The listing builds one solid part. Answer for the finished solid, in the listing's coordinates (mm). Give positions to 0.01 mm unless a question says otherwise; leave off trailing zeros. Order: outer loops, then holes, each group sorted by start corner. A loop starts at its lowest first (then second) coordinate and runs counter-clockwise, first axis right, second up. Notation, with made-up numbers: (6.5, 2) - (35.5, 2) arc R21 ccw to (35.5, 36) - close; hole circle Ø8 at (-25.5, 53.5). An arc over 180 degrees is marked (long way). Use a Markdown table: item, result. Add a question column.
1) Flat-ended cylindrical pins translate along their axes: pin 1 (1.5 mm diameter, centred on x = 31.5, y = 3, fed in from +Z); pin 2 (1 mm diameter, centred on x = 38, y = 1.5, fed in from +Z); pin 3 (10 mm diameter, centred on x = -20, y = 7, fed in from -Z). Find the tip coordinate at first contact, or state that the pin passes through.
2) Find section C-C, the plane x = 27.4. Determine the outline of the cut face in (y, z).
3) Find section A-A, the plane y = 0. Determine the outline of the cut face in (x, z).
4) Find section D-D, the plane x = -17. Determine the outline of the cut face in (y, z).
5) The mould has two halves that part along Y. Classify faces 1 (the face through (30.357, 0.931, -8.669)), 2 (the face through (107, 8.2, 0)): released by +Y, released by -Y, zero draft, split by the parting line, or undercut.
6) Straight lines are drawn through the part: line 1 (Y direction, x = -24, z = 0); line 2 (Y direction, x = 32, z = 3.25). For each, find the intervals that lie inside material, in ascending order.
7) Find section B-B, the plane z = 0. Determine the outline of the cut face in (x, y), plus the area to 3 significant figures.
from build123d import *

# Parameters (mm, degrees)
SKETCH_1_R              = 10
SKETCH_1_R_2            = 8
EXTRUDE_1_DEPTH         = 107
SKETCH_2_R              = 10
SKETCH_2_R_2            = 8
EXTRUDE_2_DEPTH         = 35.3
SKETCH2_R               = 3.1
CUT_EXTRUDE2_DEPTH      = 11
CUT_EXTRUDE2_DEPTH_BACK = 11


with BuildPart() as part:
    # 草图1 → 凸台-拉伸1 (new body)
    with BuildSketch(Plane(origin=(0, 0, 0), x_dir=(0, 0, -1), z_dir=(1, 0, 0))):
        Circle(SKETCH_1_R)
        Circle(SKETCH_1_R_2, mode=Mode.SUBTRACT)
    extrude(amount=EXTRUDE_1_DEPTH)

    # 草图2 → 凸台-拉伸2 (add)
    with BuildSketch(Plane.ZY):
        Circle(SKETCH_2_R)
        Circle(SKETCH_2_R_2, mode=Mode.SUBTRACT)
    extrude(amount=EXTRUDE_2_DEPTH)

    # Sketch2 → Cut-Extrude2 (cut, two sides)
    with BuildSketch(Plane.XY) as cut_extrude2_sk:
        with Locations((27.4, 0)):
            Circle(SKETCH2_R)
    extrude(amount=CUT_EXTRUDE2_DEPTH, mode=Mode.SUBTRACT)
    extrude(cut_extrude2_sk.sketch, amount=-CUT_EXTRUDE2_DEPTH_BACK, mode=Mode.SUBTRACT)


solid = part.part
The answers:
| question | item | result |
|---|---|---|
| 1 | pin 1 | z = 9.74 |
| 1 | pin 2 | z = 9.95 |
| 1 | pin 3 | z = -9.8 |
| 2 | outline | (-3.1, -9.51) - (-3.1, -7.37) arc R8 cw to (-3.1, 7.37) - (-3.1, 9.51) arc R10 ccw to start; (3.1, -9.51) arc R10 ccw to (3.1, 9.51) - (3.1, 7.37) arc R8 cw to (3.1, -7.37) - close |
| 3 | outline | (-35.3, -10) - (24.3, -10) - (24.3, -8) - (-35.3, -8) - close; (-35.3, 8) - (24.3, 8) - (24.3, 10) - (-35.3, 10) - close; (30.5, -10) - (107, -10) - (107, -8) - (30.5, -8) - close; (30.5, 8) - (107, 8) - (107, 10) - (30.5, 10) - close |
| 4 | outline | circle Ø20 at (0, 0); hole circle Ø16 at (0, 0) |
| 5 | face 1 | undercut |
| 5 | face 2 | zero draft |
| 6 | line 1 | -10 to -8, 8 to 10 |
| 6 | line 2 | -9.46 to -7.31, 7.31 to 9.46 |
| 7 | outline | (-35.3, -10) - (107, -10) - (107, -8) - (-35.3, -8) - close; (-35.3, 8) - (107, 8) - (107, 10) - (-35.3, 10) - close |
| 7 | area | 569 mm2 |
